Read the model definition and answer for the solid it produces. Units are mm, in the model's axes. Round coordinates to 2 decimals unless told otherwise and drop trailing zeros. Order: outer loops, then holes, each group sorted by start corner. A loop starts at its lowest first (then second) coordinate and runs counter-clockwise, first axis right, second up. Notation, with made-up numbers: (35, 25.25) -> (48, 25.25) arc R26 ccw to (48, 62.25) -> close; hole circle Ø3 at (-37.75, -27). An arc over 180 degrees is marked (long way). Use a Markdown table: item, result. Add a question column.
1. Section A-A, the plane y = 7 is taken. Give the vertices of the cut face in (x, z), then the cut area to 3 significant figures.
2. Section B-B, the plane x = 20 is taken. Give the vertices of the cut face in (y, z).
3. Given pin 1 (6 mm diameter, centred on x = 20, z = 12.5, fed in from -Y), flat-ended and moving along its own axis, determine where the tip first touches the part or whether it passes through.
4. The mould has two halves that part along X. Classify faces 1 (the face through (15, 20, 10)), 2 (the face through (0, 10, 12)), 3 (the face through (40, 10, 12)), 4 (the face through (16, 16, 9.5)): +X half, -X half, draft (parallel to the pull), parting line (faces both ways), or undercut.
5. Section C-C, the plane z = 5 is taken. Give the vertices of the cut face in (x, y).
6. Consider L1, parallel to X at y = 10, z = 17; L2, parallel to Y at x = 20, z = 6; L3, parallel to Z at x = 20, y = 15.75. Determine where each line is inside the solid, lowest interval first. Write a range as [from, to].
7. Section D-D, the plane y = 3.25 is taken. Give the vertices of the cut face in (x, z), then the cut area to 3 significant figures.
```python
from build123d import *

# Parameters (mm, degrees)
F0_W     = 40
F0_H     = 20
F1_DEPTH = 25
F2_R     = 5
F3_DEPTH = 25
F4_R     = 5
F5_DEPTH = 25


with BuildPart() as f1:
    # F0 (on Top) → F1 (new body)
    with BuildSketch(Plane.XY):
        with Locations((20, 10)):
            Rectangle(F0_W, F0_H)
    extrude(amount=F1_DEPTH)

    # F2 (on face) → F3 (cut)
    with BuildSketch(Plane.XY.offset(25)):
        with Locations((20, 10)):
            Circle(F2_R)
    extrude(amount=-F3_DEPTH, mode=Mode.SUBTRACT)

    # F4 (on face) → F5 (cut)
    with BuildSketch(Plane.XZ):
        with Locations((20, 12.5)):
            Circle(F4_R)
    extrude(amount=-F5_DEPTH, mode=Mode.SUBTRACT)


solid = f1.part
```
Verdict:
| question | item | result |
|---|---|---|
| 1 | outline | (0, 0) -> (16, 0) -> (16, 9.5) arc R5 cw to (16, 15.5) -> (16, 25) -> (0, 25) -> close; (24, 0) -> (40, 0) -> (40, 25) -> (24, 25) -> (24, 15.5) arc R5 cw to (24, 9.5) -> close |
| 1 | area | 792 mm2 |
| 2 | outline | (0, 0) -> (5, 0) -> (5, 7.5) -> (0, 7.5) -> close; (0, 17.5) -> (5, 17.5) -> (5, 25) -> (0, 25) -> close; (15, 0) -> (20, 0) -> (20, 7.5) -> (15, 7.5) -> close; (15, 17.5) -> (20, 17.5) -> (20, 25) -> (15, 25) -> close |
| 3 | pin 1 | passes through |
| 4 | face 1 | draft |
| 4 | face 2 | -X half |
| 4 | face 3 | +X half |
| 4 | face 4 | undercut |
| 5 | outline | (0, 0) -> (40, 0) -> (40, 20) -> (0, 20) -> close; hole circle Ø10 at (20, 10) |
| 6 | L1 | x = [0, 15], [25, 40] |
| 6 | L2 | y = [0, 5], [15, 20] |
| 6 | L3 | z = [0, 7.5], [17.5, 25] |
| 7 | outline | (0, 0) -> (40, 0) -> (40, 25) -> (0, 25) -> close; hole circle Ø10 at (20, 12.5) |
| 7 | area | 921 mm2 |
